Read the model definition and answer for the solid it produces. Units are mm, in the model's axes. A direction names the side the tool comes from. Round coordinates to 2 decimals unless told otherwise and drop trailing zeros. Loops run counter-clockwise (first coordinate to the right, second up) from the corner with the lowest first, then second, coordinate; pieces in that order, holes last. Notation, with made-up numbers: M -36,-34 L -14,-34 A18 ccw -14,-20 Z; hole C -18,77.5 d6. An arc over 180 degrees is marked long. Write each question's results on one line, items separated by ' | '.
from build123d import *

# Parameters (mm, degrees)
F1_DEPTH      = 5
F2_R          = 12.5
F3_DEPTH      = 30
F4_R          = 9.725
F5_DEPTH      = 29
F6_R          = 6
F7_DEPTH      = 25.4
F9_DEPTH      = 25.4
F10_R         = 4
F11_DEPTH     = 8
F12_T4_ANGLE  = 87.4800969246
F12_S5_R      = 4
F12_T6_DEPTH  = 12
F12_T10_ANGLE = 87.4800969246
F12_S11_R     = 4
F12_T12_DEPTH = 11
F12_T16_ANGLE = 87.4800969246
F12_S17_R     = 4
F12_T18_DEPTH = 11
F12_T22_ANGLE = 43.739121488
F12_S23_R     = 4
F12_T24_DEPTH = 8
F12_T28_ANGLE = 43.739121488
F12_S29_R     = 4
F12_T30_DEPTH = 8
F12_T34_ANGLE = 87.4800969246
F12_S35_R     = 4
F12_T36_DEPTH = 11
F12_T40_ANGLE = 87.4800969246
F12_S41_R     = 4
F12_T42_DEPTH = 11


# Not quite as in the source:
# - a fillet or chamfer that OpenCascade refuses, or shapes differently, is made with other operations: its cross-section is extruded or revolved along the edge and cut away or added


with BuildPart() as f1:
    # F0 (on Top) → F1 (new body)
    with BuildSketch(Plane.XY):
        Polygon((9.8149545762, 17), (-9.8149545762, 17), (-19.6299091524, 0), (-9.8149545762, -17), (9.8149545762, -17), (19.6299091524, 0), align=None)
    extrude(amount=F1_DEPTH)

    # F2 (on face) → F3 (join)
    with BuildSketch(Plane.XY.offset(5)):
        Circle(F2_R)
    extrude(amount=F3_DEPTH)

    # F4 (on face) → F5 (cut)
    with BuildSketch(Plane.XY.offset(35)):
        Circle(F4_R)
    extrude(amount=-F5_DEPTH, mode=Mode.SUBTRACT)

    # F6 (on face) → F7 (cut)
    with BuildSketch(Plane(origin=(0, 0, 0), x_dir=(1, 0, 0), z_dir=(0, 0, -1))):
        Circle(F6_R)
    extrude(amount=-F7_DEPTH, mode=Mode.SUBTRACT)

    # F8 (on face) → F9 (cut)
    with BuildSketch(Plane.XY.offset(5)):
        with BuildLine():
            ThreePointArc((-6.2749545762, 10.8685401412), (-5.5429037687, 11.6005909488), (-5.2749545762, 12.6005909488))
            ThreePointArc((-5.2749545762, 12.6005909488), (-6.2749545762, 14.3326417563), (-8.2749545762, 14.3326417563))
            Line((-8.2749545762, 14.3326417563), (-6.2749545762, 10.8685401412))
        make_face()
        with BuildLine():
            ThreePointArc((8.2749545762, 14.3326417563), (5.5429037687, 13.6005909488), (6.2749545762, 10.8685401412))
            Line((6.2749545762, 10.8685401412), (8.2749545762, 14.3326417563))
        make_face()
        with BuildLine():
            Line((8.2749545762, 14.3326417563), (6.2749545762, 10.8685401412))
            ThreePointArc((6.2749545762, 10.8685401412), (8.2749545762, 10.8685401412), (9.2749545762, 12.6005909488))
            ThreePointArc((9.2749545762, 12.6005909488), (9.0070053838, 13.6005909488), (8.2749545762, 14.3326417563))
        make_face()
        with BuildLine():
            ThreePointArc((16.5499091524, 0), (14.5499091524, 2), (12.5499091524, 0))
            Line((12.5499091524, 0), (16.5499091524, 0))
        make_face()
        with BuildLine():
            Line((16.5499091524, 0), (12.5499091524, 0))
            ThreePointArc((12.5499091524, 0), (14.5499091524, -2), (16.5499091524, 0))
        make_face()
        with BuildLine():
            ThreePointArc((9.2749545762, -12.6005909488), (8.2749545762, -10.8685401412), (6.2749545762, -10.8685401412))
            Line((6.2749545762, -10.8685401412), (8.2749545762, -14.3326417563))
            ThreePointArc((8.2749545762, -14.3326417563), (9.0070053838, -13.6005909488), (9.2749545762, -12.6005909488))
        make_face()
        with BuildLine():
            Line((8.2749545762, -14.3326417563), (6.2749545762, -10.8685401412))
            ThreePointArc((6.2749545762, -10.8685401412), (5.5429037687, -13.6005909488), (8.2749545762, -14.3326417563))
        make_face()
        with BuildLine():
            ThreePointArc((-5.2749545762, -12.6005909488), (-5.5429037687, -11.6005909488), (-6.2749545762, -10.8685401412))
            Line((-6.2749545762, -10.8685401412), (-8.2749545762, -14.3326417563))
            ThreePointArc((-8.2749545762, -14.3326417563), (-6.2749545762, -14.3326417563), (-5.2749545762, -12.6005909488))
        make_face()
        with BuildLine():
            Line((-8.2749545762, -14.3326417563), (-6.2749545762, -10.8685401412))
            ThreePointArc((-6.2749545762, -10.8685401412), (-9.0070053838, -11.6005909488), (-8.2749545762, -14.3326417563))
        make_face()
        with BuildLine():
            ThreePointArc((-16.5499091524, 0), (-14.5499091524, -2), (-12.5499091524, 0))
            Line((-12.5499091524, 0), (-16.5499091524, 0))
        make_face()
        with BuildLine():
            Line((-16.5499091524, 0), (-12.5499091524, 0))
            ThreePointArc((-12.5499091524, 0), (-14.5499091524, 2), (-16.5499091524, 0))
        make_face()
        with BuildLine():
            Line((-6.2749545762, 10.8685401412), (-8.2749545762, 14.3326417563))
            ThreePointArc((-8.2749545762, 14.3326417563), (-9.0070053838, 11.6005909488), (-6.2749545762, 10.8685401412))
        make_face()
    extrude(amount=-F9_DEPTH, mode=Mode.SUBTRACT)

    # F10 (on face) → F11 (cut)
    with BuildSketch(Plane.XY.offset(5)):
        with Locations((-7.2749545762, -12.6005909488)):
            Circle(F10_R)
        with Locations((-14.5499091524, 0)):
            Circle(F10_R)
        with Locations((-7.2749545762, 12.6005909488)):
            Circle(F10_R)
        with Locations((7.2749545762, 12.6005909488)):
            Circle(F10_R)
        with Locations((14.5499091524, 0)):
            Circle(F10_R)
        with Locations((7.2749545762, -12.6005909488)):
            Circle(F10_R)
    extrude(amount=F11_DEPTH, mode=Mode.SUBTRACT)

    # F12: fillet of radius 2.54 on 7 edges, made by hand


with BuildPart() as f12_tool2:
    # F12_s3 → F12_t4 (revolve)
    with BuildSketch(Plane(origin=(0, 0, 0), x_dir=(0, 0, 1), z_dir=(0.6913875801, -0.7224840581, 0))):
        with BuildLine():
            ThreePointArc((13, 9.96), (13.7439487758, 11.7560512242), (15.54, 12.5))
            Line((15.54, 12.5), (13, 12.5))
            Line((13, 12.5), (13, 9.96))
        make_face()
    revolve(axis=Axis((0, 0, 13), (0, 0, -1)), revolution_arc=F12_T4_ANGLE)

    # F12_s5 → F12_t6 (intersect, symmetric)
    with BuildSketch(Plane.XY.offset(15.2)):
        with Locations((-14.5499091524, 0)):
            Circle(F12_S5_R)
    extrude(amount=F12_T6_DEPTH, both=True, mode=Mode.INTERSECT)


with BuildPart() as f1_1:
    add(f1.part)

    # F12_t1: cut F12_tool2
    add(f12_tool2.part, mode=Mode.SUBTRACT)


with BuildPart() as f12_tool8:
    # F12_s9 → F12_t10 (revolve)
    with BuildSketch(Plane(origin=(0, 0, 0), x_dir=(0, 0, 1), z_dir=(0.9713833381, 0.2375171792, 0))):
        with BuildLine():
            ThreePointArc((13, 9.96), (13.7439487758, 11.7560512242), (15.54, 12.5))
            Line((15.54, 12.5), (13, 12.5))
            Line((13, 12.5), (13, 9.96))
        make_face()
    revolve(axis=Axis((0, 0, 13), (0, 0, -1)), revolution_arc=F12_T10_ANGLE)

    # F12_s11 → F12_t12 (intersect, symmetric)
    with BuildSketch(Plane.XY.offset(15.2)):
        with Locations((-7.2749545762, -12.6005909488)):
            Circle(F12_S11_R)
    extrude(amount=F12_T12_DEPTH, both=True, mode=Mode.INTERSECT)


with BuildPart() as f1_2:
    add(f1_1.part)

    # F12_t7: cut F12_tool8
    add(f12_tool8.part, mode=Mode.SUBTRACT)


with BuildPart() as f12_tool14:
    # F12_s15 → F12_t16 (revolve)
    with BuildSketch(Plane(origin=(0, 0, 0), x_dir=(0, 0, 1), z_dir=(0.2799957581, 0.9600012372, 0))):
        with BuildLine():
            ThreePointArc((13, 9.96), (13.7439487758, 11.7560512242), (15.54, 12.5))
            Line((15.54, 12.5), (13, 12.5))
            Line((13, 12.5), (13, 9.96))
        make_face()
    revolve(axis=Axis((0, 0, 13), (0, 0, -1)), revolution_arc=F12_T16_ANGLE)

    # F12_s17 → F12_t18 (intersect, symmetric)
    with BuildSketch(Plane.XY.offset(15.2)):
        with Locations((7.2749545762, -12.6005909488)):
            Circle(F12_S17_R)
    extrude(amount=F12_T18_DEPTH, both=True, mode=Mode.INTERSECT)


with BuildPart() as f1_3:
    add(f1_2.part)

    # F12_t13: cut F12_tool14
    add(f12_tool14.part, mode=Mode.SUBTRACT)


with BuildPart() as f12_tool20:
    # F12_s21 → F12_t22 (revolve)
    with BuildSketch(Plane(origin=(0, 0, 0), x_dir=(0, 0, 1), z_dir=(-0.6913758911, 0.7224952438, 0))):
        with BuildLine():
            ThreePointArc((13, 9.96), (13.7439487758, 11.7560512242), (15.54, 12.5))
            Line((15.54, 12.5), (13, 12.5))
            Line((13, 12.5), (13, 9.96))
        make_face()
    revolve(axis=Axis((0, 0, 13), (0, 0, -1)), revolution_arc=F12_T22_ANGLE)

    # F12_s23 → F12_t24 (intersect, symmetric)
    with BuildSketch(Plane.XY.offset(15.2)):
        with Locations((14.5499091524, 0)):
            Circle(F12_S23_R)
    extrude(amount=F12_T24_DEPTH, both=True, mode=Mode.INTERSECT)


with BuildPart() as f1_4:
    add(f1_3.part)

    # F12_t19: cut F12_tool20
    add(f12_tool20.part, mode=Mode.SUBTRACT)


with BuildPart() as f12_tool26:
    # F12_s27 → F12_t28 (revolve)
    with BuildSketch(Plane.XZ):
        with BuildLine():
            ThreePointArc((9.96, 13), (11.7560512242, 13.7439487758), (12.5, 15.54))
            Line((12.5, 15.54), (12.5, 13))
            Line((12.5, 13), (9.96, 13))
        make_face()
    revolve(axis=Axis((0, 0, 13), (0, 0, -1)), revolution_arc=F12_T28_ANGLE)

    # F12_s29 → F12_t30 (intersect, symmetric)
    with BuildSketch(Plane.XY.offset(15.2)):
        with Locations((14.5499091524, 0)):
            Circle(F12_S29_R)
    extrude(amount=F12_T30_DEPTH, both=True, mode=Mode.INTERSECT)


with BuildPart() as f1_5:
    add(f1_4.part)

    # F12_t25: cut F12_tool26
    add(f12_tool26.part, mode=Mode.SUBTRACT)


with BuildPart() as f12_tool32:
    # F12_s33 → F12_t34 (revolve)
    with BuildSketch(Plane(origin=(0, 0, 0), x_dir=(0, 0, 1), z_dir=(-0.9713833381, -0.2375171792, 0))):
        with BuildLine():
            ThreePointArc((13, 9.96), (13.7439487758, 11.7560512242), (15.54, 12.5))
            Line((15.54, 12.5), (13, 12.5))
            Line((13, 12.5), (13, 9.96))
        make_face()
    revolve(axis=Axis((0, 0, 13), (0, 0, -1)), revolution_arc=F12_T34_ANGLE)

    # F12_s35 → F12_t36 (intersect, symmetric)
    with BuildSketch(Plane.XY.offset(15.2)):
        with Locations((7.2749545762, 12.6005909488)):
            Circle(F12_S35_R)
    extrude(amount=F12_T36_DEPTH, both=True, mode=Mode.INTERSECT)


with BuildPart() as f1_6:
    add(f1_5.part)

    # F12_t31: cut F12_tool32
    add(f12_tool32.part, mode=Mode.SUBTRACT)


with BuildPart() as f12_tool38:
    # F12_s39 → F12_t40 (revolve)
    with BuildSketch(Plane(origin=(0, 0, 0), x_dir=(0, 0, 1), z_dir=(-0.2799957581, -0.9600012372, 0))):
        with BuildLine():
            ThreePointArc((13, 9.96), (13.7439487758, 11.7560512242), (15.54, 12.5))
            Line((15.54, 12.5), (13, 12.5))
            Line((13, 12.5), (13, 9.96))
        make_face()
    revolve(axis=Axis((0, 0, 13), (0, 0, -1)), revolution_arc=F12_T40_ANGLE)

    # F12_s41 → F12_t42 (intersect, symmetric)
    with BuildSketch(Plane.XY.offset(15.2)):
        with Locations((-7.2749545762, 12.6005909488)):
            Circle(F12_S41_R)
    extrude(amount=F12_T42_DEPTH, both=True, mode=Mode.INTERSECT)


with BuildPart() as f1_7:
    add(f1_6.part)

    # F12_t37: cut F12_tool38
    add(f12_tool38.part, mode=Mode.SUBTRACT)


solid = f1_7.part
Item 1: Straight lines are drawn through the part: line 1 (Y direction, x = 0, z = 3.8); line 2 (X direction, y = 14, z = 4); line 3 (Z direction, x = 8.5, y = -10). For each, find the intervals that lie inside material, in ascending order.
Outcome:
line 1: y = -17 to -6, 6 to 17 | line 2: x = -11.55 to -8.7, -5.85 to 5.85, 8.7 to 11.55 | line 3: z = 0 to 5
Item 2: The part is cut by section B-B (z = 3.5). Determine the outline of the cut face in (x, y), plus the area to 3 significant figures.
Outcome:
outline: M -19.63,0 L -9.81,-17 L 9.81,-17 L 19.63,0 L 9.81,17 L -9.81,17 Z; hole C -14.55,0 d4; hole C -7.27,-12.6 d4; hole C -7.27,12.6 d4; hole C 0,0 d12; hole C 7.27,-12.6 d4; hole C 7.27,12.6 d4; hole C 14.55,0 d4 | area: 813 mm2
Item 3: Flat-ended cylindrical pins translate along their axes: pin 1 (6 mm diameter, centred on x = -11.5, z = 31.5, fed in from +Y); pin 2 (2 mm diameter, centred on y = 6.5, z = 9, fed in from +X) (3 decimals); pin 3 (6 mm diameter, centred on y = 5, z = 12, fed in from +X); pin 4 (9.5 mm diameter, centred on x = 0, y = 0, fed in from +Z). Find the tip coordinate at first contact, or state that the pin passes through.
Outcome:
pin 1: stops at y = 9.17 | pin 2: stops at x = 11.225 | pin 3: stops at x = 12.09 | pin 4: passes through
Item 4: The part is cut by section D-D (y = 13.5). Determine the outline of the cut face in (x, z).
Outcome:
outline: M -11.84,0 L -9.06,0 L -9.06,5 L -11.84,5 Z; M -5.49,0 L 5.49,0 L 5.49,5 L -5.49,5 Z; M 9.06,0 L 11.84,0 L 11.84,5 L 9.06,5 Z
Item 5: The part is cut by section C-C (z = 19.5). Determine the outline of the cut face in (x, y) (3 decimals), plus the area to 3 significant figures.
Outcome:
outline: C 0,0 d25; hole C 0,0 d19.45 | area: 194 mm2
Item 6: For faces 4 (the face through (5.231, 9.162, 9.025)), 5 (the face through (4, 12, 5)), 6 (the face through (4.2, 4.5, 6)), determine the directions among +Z, -Z, +X, -X, +Y, -Y from which every point of the face is accessible in a straight line to the end or side of a thin tool.
Outcome:
face 4: +Y | face 5: none | face 6: +Z
Item 7: The mould has two halves that part along X. Classify faces 1 (the face through (11.547, -4.788, 19.79)), 2 (the face through (-5.32, 9.11, 9.03)), 3 (the face through (-14.654, 8.619, 2.465)): pulls with the +X half, pulls with the -X half, needs draft (parallel to the pull), parting line crosses it, or undercut.
Outcome:
face 1: parting line crosses it | face 2: undercut | face 3: pulls with the -X half
Item 8: The part is cut by section A-A (x = 0). Determine the outline of the cut face in (y, z) (3 decimals).
Outcome:
outline: M -17,0 L -6,0 L -6,6 L -9.725,6 L -9.725,35 L -12.5,35 L -12.5,5 L -17,5 Z; M 6,0 L 17,0 L 17,5 L 12.5,5 L 12.5,35 L 9.725,35 L 9.725,6 L 6,6 Z
